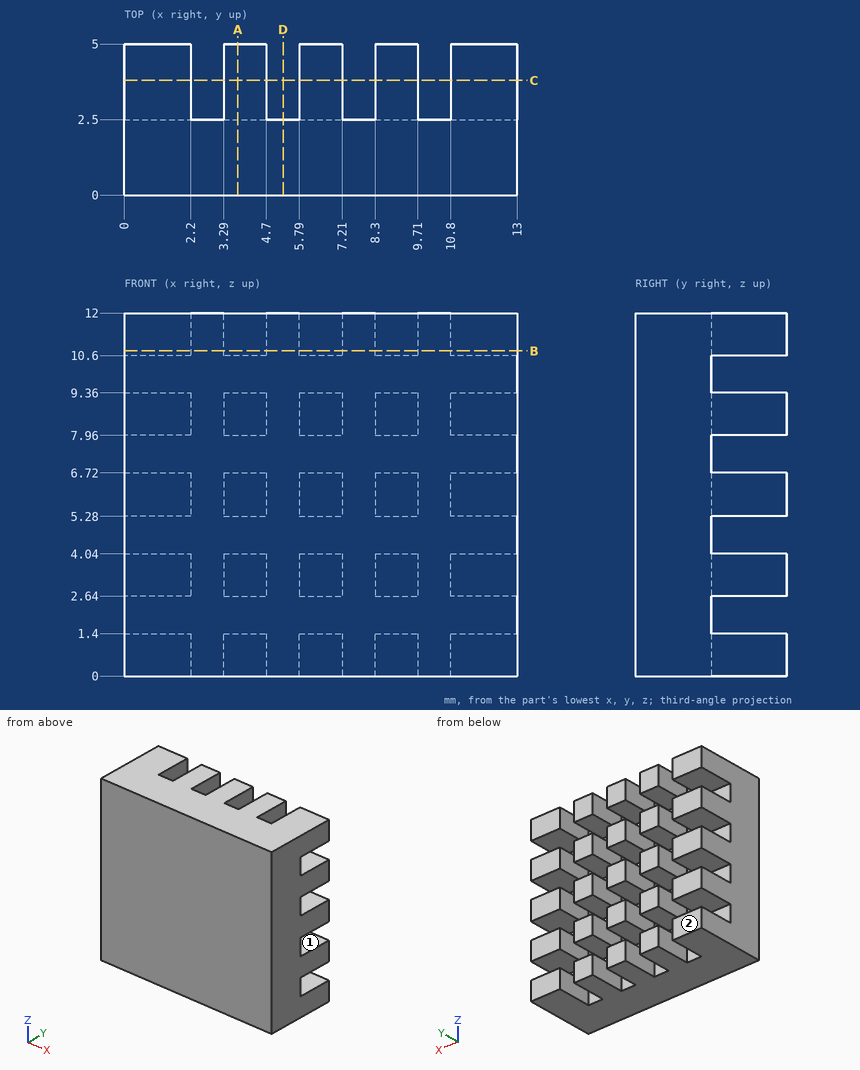
The figure shows three views and two pictorial views of one solid part (mm, origin at its lowest corner). Answer the questions. A direction names the side the tool comes from. Round coordinates to 2 decimals unless told otherwise and drop trailing zeros. Order: outer loops, then holes, each group sorted by start corner. A loop starts at its lowest first (then second) coordinate and runs counter-clockwise, first axis right, second up.
Q1. A tool of negligible diameter and unlimited length cuts with its end or side. For the marked faces 1 and 2, from which of +Z, -Z, +X, -X, +Y, -Y can it reach the whole face along a straight path? Write none if from no direction.
Solution:
face 1: +X, -X, +Y
face 2: +Z, -Z, +X, -X, +Y
Q2. Find the intervals of material crossed by line 1 along X through (y, z) = (4.4, 6.25); line 2 along Z through (x, y) = (4, 3.6); line 3 along Y through (x, z) = (7.75, 6.5), in increasing order.
Solution:
line 1: x = 0 to 2.2, 3.29 to 4.7, 5.79 to 7.21, 8.3 to 9.71, 10.8 to 13
line 2: z = 0 to 1.4, 2.64 to 4.04, 5.28 to 6.72, 7.96 to 9.36, 10.6 to 12
line 3: y = 0 to 2.5
Q3. A cutting plane is placed at C-C, the plane y = 3.8. Count the separate pieces of the cut face and the enclosed holes in it, then the cut area to 3 significant figures.
Solution:
separate pieces: 25
enclosed holes: 0
area: 60.8 mm2
Q4. A cutting plane is placed at A-A, the plane x = 3.75. Determine the outline of the cut face in (y, z), then the cut area to 3 significant figures.
Solution:
outline: (0, 0) - (5, 0) - (5, 1.4) - (2.5, 1.4) - (2.5, 2.64) - (5, 2.64) - (5, 4.04) - (2.5, 4.04) - (2.5, 5.28) - (5, 5.28) - (5, 6.72) - (2.5, 6.72) - (2.5, 7.96) - (5, 7.96) - (5, 9.36) - (2.5, 9.36) - (2.5, 10.6) - (5, 10.6) - (5, 12) - (0, 12) - close
area: 47.6 mm2
Q5. A cutting plane is placed at B-B, the plane z = 10.75. Determine the outline of the cut face in (x, y).
Solution:
outline: (0, 0) - (13, 0) - (13, 5) - (10.8, 5) - (10.8, 2.5) - (9.71, 2.5) - (9.71, 5) - (8.3, 5) - (8.3, 2.5) - (7.21, 2.5) - (7.21, 5) - (5.79, 5) - (5.79, 2.5) - (4.7, 2.5) - (4.7, 5) - (3.29, 5) - (3.29, 2.5) - (2.2, 2.5) - (2.2, 5) - (0, 5) - close
Q6. A cutting plane is placed at D-D, the plane x = 5.25. Determine the outline of the cut face in (y, z).
Solution:
outline: (0, 0) - (2.5, 0) - (2.5, 12) - (0, 12) - close
